The drawing under review shows one solid part. Ordinate dimensions are in mm from its lowest x, y, z. A direction names the side the tool comes from. Give positions to 0.01 mm unless a question says otherwise; leave off trailing zeros. Order: outer loops, then holes, each group sorted by start corner. A loop starts at its lowest first (then second) coordinate and runs counter-clockwise, first axis right, second up. Notation, with made-up numbers: M -26.75,-4 L -18.75,-4 A28 ccw -18.75,24 Z; hole C 31,58 d6. An arc over 180 degrees is marked long. Put each result on its own line as item: value. Start each with the question number.
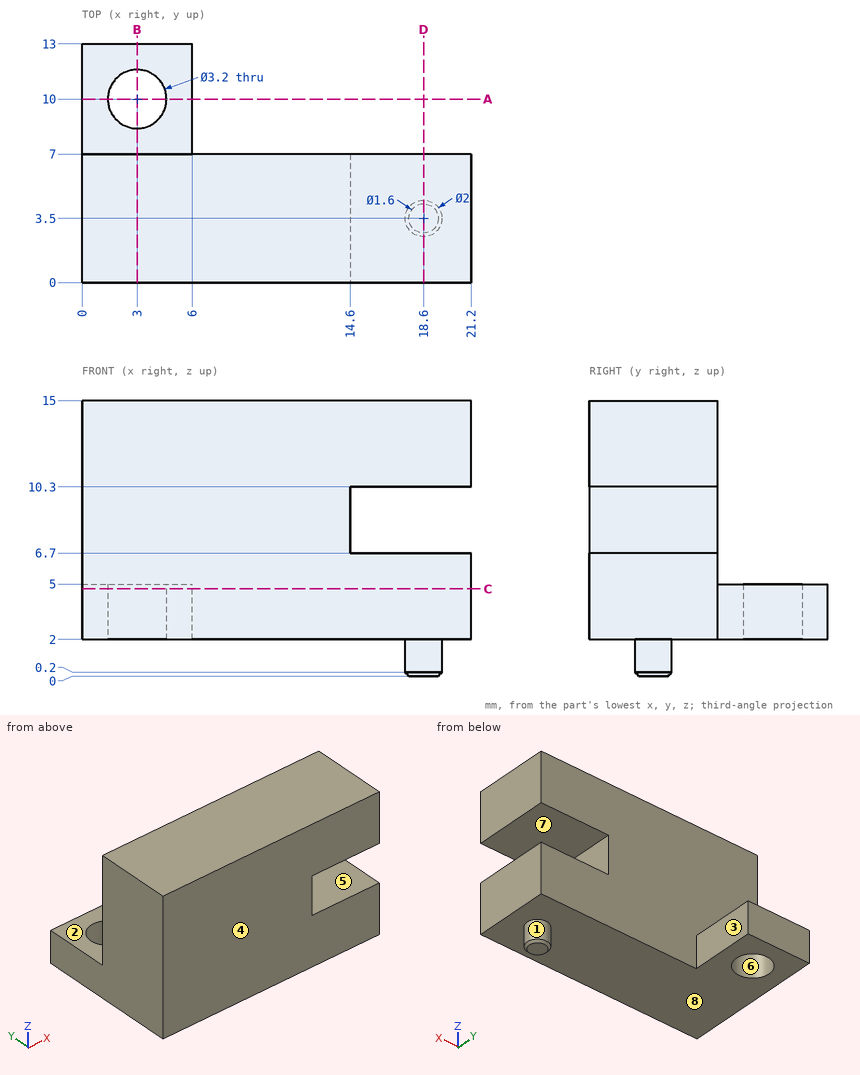
1. Consider section D-D on x = 18.6. Give the boundary of the cut face in (y, z), then the cut area to 3 significant figures.
2. The part is to be moulded in two halves that separate along Z. For the marked faces 6, 7 and 8, say which applies: +Z half, -Z half, draft (parallel to the pull), parting line (faces both ways), or undercut.
3. Machinability: for the marked faces 1, 2, 3, 4 and 5, which of the approach directions +Z, -Z, +X, -X, +Y, -Y give a long, thin tool a straight path to every point of the face, cutting with its end or side? Answer none if there is none.
4. Consider section A-A on y = 10. Give the boundary of the cut face in (x, z).
5. Consider section B-B on x = 3. Give the boundary of the cut face in (y, z).
6. Consider section C-C on z = 4.75. Give the boundary of the cut face in (x, y), then the cut area to 3 significant figures.
7. Insertion check: pin 1 (1.5 mm diameter, centred on x = 13, y = 8.5, fed in from -Z); pin 2 (3 mm diameter, centred on y = 1.5, z = 5.5, fed in from -X); pin 3 (6.5 mm diameter, centred on x = 5.5, z = 10, fed in from +Y); pin 4 (5 mm diameter, centred on x = 3, y = 10, fed in from -Z). Each pin has a flat end and moves straight along its axis. Give the tip position at first contact, or say it passes through.
8. To check wall thickness, follow probe 1 along Y at (x, z) = (3, 2.9); probe 2 along Z at (x, y) = (19.75, 3.5); probe 3 along Y at (x, z) = (12.75, 4). State the ranges of each line that lie inside material, in increasing order.
Returned:
1. outline: M 0,2 L 2.5,2 L 2.5,0.2 L 2.7,0 L 4.3,0 L 4.5,0.2 L 4.5,2 L 7,2 L 7,6.7 L 0,6.7 Z; M 0,10.3 L 7,10.3 L 7,15 L 0,15 Z
1. area: 69.8 mm2
2. face 6: draft
2. face 7: undercut
2. face 8: -Z half
3. face 1: -Z
3. face 2: +Z, +X, -X, +Y
3. face 3: +Z, -Z, +X, +Y
3. face 4: +Z, -Z, +X, -X, -Y
3. face 5: +X, +Y, -Y
4. outline: M 0,2 L 1.4,2 L 1.4,5 L 0,5 Z; M 4.6,2 L 6,2 L 6,5 L 4.6,5 Z
5. outline: M 0,2 L 8.4,2 L 8.4,5 L 7,5 L 7,15 L 0,15 Z; M 11.6,2 L 13,2 L 13,5 L 11.6,5 Z
6. outline: M 0,0 L 21.2,0 L 21.2,7 L 6,7 L 6,13 L 0,13 Z; hole C 3,10 d3.2
6. area: 176 mm2
7. pin 1: passes through
7. pin 2: stops at x = 0
7. pin 3: stops at y = 7
7. pin 4: stops at z = 2
8. probe 1: y = 0 to 8.4, 11.6 to 13
8. probe 2: z = 2 to 6.7, 10.3 to 15
8. probe 3: y = 0 to 7
